Can you work these out from the model? Positions are in its coordinate system, mm. A direction names the side the tool comes from. Give positions to 0.01 mm unless a question says otherwise; leave off trailing zeros. Answer as CSV lines item,"result".
```python
from build123d import *

# Parameters (mm, degrees)
SKETCH1_R           = 2.1463
BOSS_EXTRUDE1_DEPTH = 115


with BuildPart() as part:
    # Sketch1 → Boss-Extrude1 (new body, symmetric)
    with BuildSketch(Plane.XY):
        with BuildLine():
            Line((-19.9898, 7.9883), (-19.9898, 3.2893))
            ThreePointArc((-19.9898, 3.2893), (-19.75917588, 2.73252412), (-19.2024, 2.5019))
            Line((-19.2024, 2.5019), (-18.4912, 2.5019))
            ThreePointArc((-18.4912, 2.5019), (-18.275673853, 2.591173853), (-18.1864, 2.8067))
            Line((-18.1864, 2.8067), (-18.1864, 4.9149))
            ThreePointArc((-18.1864, 4.9149), (-17.668965253, 5.689295824), (-16.755503096, 5.507596904))
            Line((-16.755503096, 5.507596904), (-14.500665747, 3.252759555))
            ThreePointArc((-14.500665747, 3.252759555), (-13.850954457, 2.280397894), (-13.622806192, 1.133419111))
            Line((-13.622806192, 1.133419111), (-13.622806192, -1.133419111))
            ThreePointArc((-13.622806192, -1.133419111), (-13.850954457, -2.280397894), (-14.500665747, -3.252759555))
            Line((-14.500665747, -3.252759555), (-16.755503096, -5.507596904))
            ThreePointArc((-16.755503096, -5.507596904), (-17.668965253, -5.689295824), (-18.1864, -4.9149))
            Line((-18.1864, -4.9149), (-18.1864, -2.8067))
            ThreePointArc((-18.1864, -2.8067), (-18.275673853, -2.591173853), (-18.4912, -2.5019))
            Line((-18.4912, -2.5019), (-19.2024, -2.5019))
            ThreePointArc((-19.2024, -2.5019), (-19.75917588, -2.73252412), (-19.9898, -3.2893))
            Line((-19.9898, -3.2893), (-19.9898, -7.9883))
            ThreePointArc((-19.9898, -7.9883), (-19.402080467, -9.407180467), (-17.9832, -9.9949))
            Line((-17.9832, -9.9949), (-13.2842, -9.9949))
            ThreePointArc((-13.2842, -9.9949), (-12.72742412, -9.76427588), (-12.4968, -9.2075))
            Line((-12.4968, -9.2075), (-12.4968, -8.4963))
            ThreePointArc((-12.4968, -8.4963), (-12.586073853, -8.280773853), (-12.8016, -8.1915))
            Line((-12.8016, -8.1915), (-14.9098, -8.1915))
            ThreePointArc((-14.9098, -8.1915), (-15.684195824, -7.674065253), (-15.502496904, -6.760603096))
            Line((-15.502496904, -6.760603096), (-13.247659555, -4.505765747))
            ThreePointArc((-13.247659555, -4.505765747), (-12.275297894, -3.856054457), (-11.128319111, -3.627906192))
            Line((-11.128319111, -3.627906192), (-8.861480889, -3.627906192))
            ThreePointArc((-8.861480889, -3.627906192), (-7.714502106, -3.856054457), (-6.742140445, -4.505765747))
            Line((-6.742140445, -4.505765747), (-4.487303096, -6.760603096))
            ThreePointArc((-4.487303096, -6.760603096), (-4.305604176, -7.674065253), (-5.08, -8.1915))
            Line((-5.08, -8.1915), (-7.1882, -8.1915))
            ThreePointArc((-7.1882, -8.1915), (-7.403726147, -8.280773853), (-7.493, -8.4963))
            Line((-7.493, -8.4963), (-7.493, -9.2075))
            ThreePointArc((-7.493, -9.2075), (-7.26237588, -9.76427588), (-6.7056, -9.9949))
            Line((-6.7056, -9.9949), (0, -9.9949))
            Line((0, -9.9949), (6.7056, -9.9949))
            ThreePointArc((6.7056, -9.9949), (7.26237588, -9.76427588), (7.493, -9.2075))
            Line((7.493, -9.2075), (7.493, -8.4963))
            ThreePointArc((7.493, -8.4963), (7.403726147, -8.280773853), (7.1882, -8.1915))
            Line((7.1882, -8.1915), (5.08, -8.1915))
            ThreePointArc((5.08, -8.1915), (4.305604176, -7.674065253), (4.487303096, -6.760603096))
            Line((4.487303096, -6.760603096), (6.742140445, -4.505765747))
            ThreePointArc((6.742140445, -4.505765747), (7.714502106, -3.856054457), (8.861480889, -3.627906192))
            Line((8.861480889, -3.627906192), (11.128319111, -3.627906192))
            ThreePointArc((11.128319111, -3.627906192), (12.275297894, -3.856054457), (13.247659555, -4.505765747))
            Line((13.247659555, -4.505765747), (15.502496904, -6.760603096))
            ThreePointArc((15.502496904, -6.760603096), (15.684195824, -7.674065253), (14.9098, -8.1915))
            Line((14.9098, -8.1915), (12.8016, -8.1915))
            ThreePointArc((12.8016, -8.1915), (12.586073853, -8.280773853), (12.4968, -8.4963))
            Line((12.4968, -8.4963), (12.4968, -9.2075))
            ThreePointArc((12.4968, -9.2075), (12.72742412, -9.76427588), (13.2842, -9.9949))
            Line((13.2842, -9.9949), (17.9832, -9.9949))
            ThreePointArc((17.9832, -9.9949), (19.402080467, -9.407180467), (19.9898, -7.9883))
            Line((19.9898, -7.9883), (19.9898, -3.2893))
            ThreePointArc((19.9898, -3.2893), (19.75917588, -2.73252412), (19.2024, -2.5019))
            Line((19.2024, -2.5019), (18.4912, -2.5019))
            ThreePointArc((18.4912, -2.5019), (18.275673853, -2.591173853), (18.1864, -2.8067))
            Line((18.1864, -2.8067), (18.1864, -4.9149))
            ThreePointArc((18.1864, -4.9149), (17.668965253, -5.689295824), (16.755503096, -5.507596904))
            Line((16.755503096, -5.507596904), (14.500665747, -3.252759555))
            ThreePointArc((14.500665747, -3.252759555), (13.850954457, -2.280397894), (13.622806192, -1.133419111))
            Line((13.622806192, -1.133419111), (13.622806192, 1.133419111))
            ThreePointArc((13.622806192, 1.133419111), (13.850954457, 2.280397894), (14.500665747, 3.252759555))
            Line((14.500665747, 3.252759555), (16.755503096, 5.507596904))
            ThreePointArc((16.755503096, 5.507596904), (17.668965253, 5.689295824), (18.1864, 4.9149))
            Line((18.1864, 4.9149), (18.1864, 2.8067))
            ThreePointArc((18.1864, 2.8067), (18.275673853, 2.591173853), (18.4912, 2.5019))
            Line((18.4912, 2.5019), (19.2024, 2.5019))
            ThreePointArc((19.2024, 2.5019), (19.75917588, 2.73252412), (19.9898, 3.2893))
            Line((19.9898, 3.2893), (19.9898, 7.9883))
            ThreePointArc((19.9898, 7.9883), (19.402080467, 9.407180467), (17.9832, 9.9949))
            Line((17.9832, 9.9949), (13.2842, 9.9949))
            ThreePointArc((13.2842, 9.9949), (12.72742412, 9.76427588), (12.4968, 9.2075))
            Line((12.4968, 9.2075), (12.4968, 8.4963))
            ThreePointArc((12.4968, 8.4963), (12.586073853, 8.280773853), (12.8016, 8.1915))
            Line((12.8016, 8.1915), (14.9098, 8.1915))
            ThreePointArc((14.9098, 8.1915), (15.684195824, 7.674065253), (15.502496904, 6.760603096))
            Line((15.502496904, 6.760603096), (13.247659555, 4.505765747))
            ThreePointArc((13.247659555, 4.505765747), (12.275297894, 3.856054457), (11.128319111, 3.627906192))
            Line((11.128319111, 3.627906192), (8.861480889, 3.627906192))
            ThreePointArc((8.861480889, 3.627906192), (7.714502106, 3.856054457), (6.742140445, 4.505765747))
            Line((6.742140445, 4.505765747), (4.487303096, 6.760603096))
            ThreePointArc((4.487303096, 6.760603096), (4.305604176, 7.674065253), (5.08, 8.1915))
            Line((5.08, 8.1915), (7.1882, 8.1915))
            ThreePointArc((7.1882, 8.1915), (7.403726147, 8.280773853), (7.493, 8.4963))
            Line((7.493, 8.4963), (7.493, 9.2075))
            ThreePointArc((7.493, 9.2075), (7.26237588, 9.76427588), (6.7056, 9.9949))
            Line((6.7056, 9.9949), (0, 9.9949))
            Line((0, 9.9949), (-6.7056, 9.9949))
            ThreePointArc((-6.7056, 9.9949), (-7.26237588, 9.76427588), (-7.493, 9.2075))
            Line((-7.493, 9.2075), (-7.493, 8.4963))
            ThreePointArc((-7.493, 8.4963), (-7.403726147, 8.280773853), (-7.1882, 8.1915))
            Line((-7.1882, 8.1915), (-5.08, 8.1915))
            ThreePointArc((-5.08, 8.1915), (-4.305604176, 7.674065253), (-4.487303096, 6.760603096))
            Line((-4.487303096, 6.760603096), (-6.742140445, 4.505765747))
            ThreePointArc((-6.742140445, 4.505765747), (-7.714502106, 3.856054457), (-8.861480889, 3.627906192))
            Line((-8.861480889, 3.627906192), (-11.128319111, 3.627906192))
            ThreePointArc((-11.128319111, 3.627906192), (-12.275297894, 3.856054457), (-13.247659555, 4.505765747))
            Line((-13.247659555, 4.505765747), (-15.502496904, 6.760603096))
            ThreePointArc((-15.502496904, 6.760603096), (-15.684195824, 7.674065253), (-14.9098, 8.1915))
            Line((-14.9098, 8.1915), (-12.8016, 8.1915))
            ThreePointArc((-12.8016, 8.1915), (-12.586073853, 8.280773853), (-12.4968, 8.4963))
            Line((-12.4968, 8.4963), (-12.4968, 9.2075))
            ThreePointArc((-12.4968, 9.2075), (-12.72742412, 9.76427588), (-13.2842, 9.9949))
            Line((-13.2842, 9.9949), (-17.9832, 9.9949))
            ThreePointArc((-17.9832, 9.9949), (-19.402080467, 9.407180467), (-19.9898, 7.9883))
        make_face()
        with Locations((-9.9949, 0)):
            Circle(SKETCH1_R, mode=Mode.SUBTRACT)
        with Locations((9.9949, 0)):
            Circle(SKETCH1_R, mode=Mode.SUBTRACT)
        with BuildLine():
            Line((-6.366993808, 1.133419111), (-6.366993808, -1.133419111))
            ThreePointArc((-6.366993808, -1.133419111), (-6.138845543, -2.280397894), (-5.489134253, -3.252759555))
            Line((-5.489134253, -3.252759555), (-0.939581002, -7.802312806))
            ThreePointArc((-0.939581002, -7.802312806), (0, -8.1915), (0.939581002, -7.802312806))
            Line((0.939581002, -7.802312806), (5.489134253, -3.252759555))
            ThreePointArc((5.489134253, -3.252759555), (6.138845543, -2.280397894), (6.366993808, -1.133419111))
            Line((6.366993808, -1.133419111), (6.366993808, 1.133419111))
            ThreePointArc((6.366993808, 1.133419111), (6.138845543, 2.280397894), (5.489134253, 3.252759555))
            Line((5.489134253, 3.252759555), (0.939581002, 7.802312806))
            ThreePointArc((0.939581002, 7.802312806), (0, 8.1915), (-0.939581002, 7.802312806))
            Line((-0.939581002, 7.802312806), (-5.489134253, 3.252759555))
            ThreePointArc((-5.489134253, 3.252759555), (-6.138845543, 2.280397894), (-6.366993808, 1.133419111))
        make_face(mode=Mode.SUBTRACT)
    extrude(amount=BOSS_EXTRUDE1_DEPTH, both=True)


solid = part.part
```
Item 1: For pin 1 (0.7 mm diameter, centred on x = 10, z = -14, fed in from +Y); pin 2 (0.6 mm diameter, centred on x = -18.5, z = 38, fed in from -Y); pin 3 (12 mm diameter, centred on x = 11.5, z = 62.5, fed in from +Y); pin 4 (0.6 mm diameter, centred on y = 9, z = 24, fed in from -X), each with a flat end and sliding along its axis, tell me the tip position at first contact or that it passes through.
Numbers:
pin 1,"stops at y = 3.63"
pin 2,"stops at y = -9.98"
pin 3,"stops at y = 9.99"
pin 4,"stops at x = -19.86"
Item 2: Please list where these lines run through material, in increasing order: line 1 along Y through (x, z) = (-14.5, 105.5); line 2 along Y through (x, z) = (-3, 88.5); line 3 along Y through (x, z) = (2, -58).
Numbers:
line 1,"y = -9.99 to -8.19, -5.76 to -3.25, 3.25 to 5.76, 8.19 to 9.99"
line 2,"y = -9.99 to -5.74, 5.74 to 9.99"
line 3,"y = -9.99 to -6.74, 6.74 to 9.99"
Item 3: We'd pull the mould along Y, two halves only. Please class faces 3 (the flat face through (3.18, -5.56, 1.61)), 4 (the flat face through (0, 9.995, 2)), 5 (the flat face through (-5, -4, -115)): released by +Y, released by -Y, zero draft, split by the parting line, or undercut.
Numbers:
face 3,"undercut"
face 4,"released by +Y"
face 5,"zero draft"
Item 4: For faces 1 (the flat face through (0, -9.995, 2)), 2 (the flat face through (-3.18, 5.56, 1.61)), which set-ups out of +Z, -Z, +X, -X, +Y, -Y let a thin tool reach every point of the face, with its end or its side?
Numbers:
face 1,"+Z, -Z, +X, -X, -Y"
face 2,"+Z, -Z"
Item 5: Imagine slicing it at A-A, the plane z = 14. Give the number of separate pieces and of enclosed holes in the cut face, then the cut area to 4 significant figures.
Numbers:
separate pieces,"1"
enclosed holes,"3"
area,"328.5 mm²"
